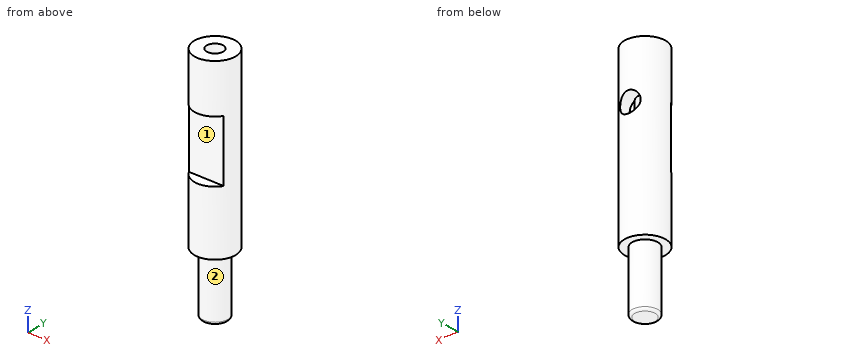
```python
from build123d import *

# Parameters (mm, degrees)
SKETCH1_R                      = 2.5
BOSS_EXTRUDE1_DEPTH            = 12
SKETCH2_R                      = 4
BOSS_EXTRUDE2_DEPTH            = 34
F_3_2_3_2_DIAMETER_HOLE1_D     = 3.2
F_3_2_3_2_DIAMETER_HOLE1_DEPTH = 13.03862301
F_3_2_3_2_DIAMETER_HOLE1_TIP   = 0.96137699
CUT_EXTRUDE1_DEPTH             = 35.467375879
CUT_EXTRUDE1_DEPTH_BACK        = 35.467375879
SKETCH6_W                      = 12
SKETCH6_H                      = 2
F_4_0_4_DIAMETER_HOLE3_D       = 4
F_4_0_4_DIAMETER_HOLE3_DEPTH   = 2.798278762
F_4_0_4_DIAMETER_HOLE3_TIP     = 1.201721238
FILLET1_R                      = 0.5


with BuildPart() as part:
    # Sketch1 → Boss-Extrude1 (new body)
    with BuildSketch(Plane.XY):
        Circle(SKETCH1_R)
    extrude(amount=-BOSS_EXTRUDE1_DEPTH)

    # Sketch2 → Boss-Extrude2 (add)
    with BuildSketch(Plane.XY):
        Circle(SKETCH2_R)
    extrude(amount=BOSS_EXTRUDE2_DEPTH)

    # Ø3.2 (3.2) Diameter Hole1
    with Locations(Plane.XY.offset(34)):
        with Locations((0, 0)):
            Hole(F_3_2_3_2_DIAMETER_HOLE1_D / 2, depth=F_3_2_3_2_DIAMETER_HOLE1_DEPTH)
            with Locations((0, 0, -(F_3_2_3_2_DIAMETER_HOLE1_DEPTH + F_3_2_3_2_DIAMETER_HOLE1_TIP / 2))):  # 118° drill point
                Cone(0, F_3_2_3_2_DIAMETER_HOLE1_D / 2, F_3_2_3_2_DIAMETER_HOLE1_TIP, mode=Mode.SUBTRACT)

    # Sketch6 → Cut-Extrude1 (cut, two sides: drawn at the far end of the back side and taken through both)
    with BuildSketch(Plane(origin=(0, 0, 0), x_dir=(0, 0, -1), z_dir=(1, 0, 0)).offset(-CUT_EXTRUDE1_DEPTH_BACK)):
        with Locations((-18.5, -3)):
            Rectangle(SKETCH6_W, SKETCH6_H)
    extrude(amount=CUT_EXTRUDE1_DEPTH + CUT_EXTRUDE1_DEPTH_BACK, mode=Mode.SUBTRACT)

    # Ø4.0 (4) Diameter Hole3
    with Locations(Plane(origin=(-0.101557348, 3.998710555, 23.218070674), x_dir=(0.999677638825, 0.025389337009, 0), z_dir=(-0.025389337009, 0.999677638825, 0))):
        with Locations((0, 0)):
            Hole(F_4_0_4_DIAMETER_HOLE3_D / 2, depth=F_4_0_4_DIAMETER_HOLE3_DEPTH)
            with Locations((0, 0, -(F_4_0_4_DIAMETER_HOLE3_DEPTH + F_4_0_4_DIAMETER_HOLE3_TIP / 2))):  # 118° drill point
                Cone(0, F_4_0_4_DIAMETER_HOLE3_D / 2, F_4_0_4_DIAMETER_HOLE3_TIP, mode=Mode.SUBTRACT)

    # Fillet1
    fillet1_edges = [part.edges().sort_by_distance(p)[0] for p in [
        (-2.5, 0, -12),
    ]]
    fillet(fillet1_edges, radius=FILLET1_R)


solid = part.part
```
Geometry check sheet. Reference: the model listing, model coordinates, mm. Face numbers are marked on the shaded views. Give positions to 0.01 mm unless a question says otherwise; leave off trailing zeros. Order: outer loops, then holes, each group sorted by start corner. A loop starts at its lowest first (then second) coordinate and runs counter-clockwise, first axis right, second up.
1. Section check D-D, the plane z = 4.5. Enter the section's corners in (x, y).
2. Thickness scan on L1, parallel to Y at x = 0, z = 26.5; L2, parallel to Y at x = -1.5, z = -6; L3, parallel to Z at x = 3, y = 1.75. Record the ranges inside material, lowest first.
3. Gauge pin test, flat ends, axial feed: pin 1 Ø0.6 at (x, y) = (-0.5, -3.5) entering from -Z; pin 2 Ø1 at (y, z) = (-1, 17.5) entering from +X; pin 3 Ø2.5 at (x, y) = (0, 0) entering from +Z. Record the tip position at first contact, or that the pin passes through.
4. Release check for a two-part mould opening along Z. For the marked faces 1 and 2 record: pulls with the +Z half, pulls with the -Z half, needs draft (parallel to the pull), parting line crosses it, or undercut.
5. Section check B-B, the plane z = 19.5. Enter the section's corners in (x, y), and give its area (3 significant figures).
6. Section check A-A, the plane y = -3.25. Enter the section's corners in (x, z), and give its area (3 significant figures).
7. Section check C-C, the plane z = -4. Enter the section's corners in (x, y).
Values follow:
1. outline: circle Ø8 at (0, 0)
2. L1: y = -4 to -1.6, 1.6 to 4
2. L2: y = -2 to 2
2. L3: z = 0 to 34
3. pin 1: stops at z = 0
3. pin 2: stops at x = 3.97
3. pin 3: stops at z = 20.75
4. face 1: undercut
4. face 2: needs draft
5. outline: (-3.46, -2) - (3.46, -2) arc R4 ccw (long way) to start
5. area: 40.4 mm2
6. outline: (-2.33, 0) - (2.33, 0) - (2.33, 12.5) - (-2.33, 12.5) - close; (-2.33, 24.5) - (2.33, 24.5) - (2.33, 34) - (-2.33, 34) - close
6. area: 103 mm2
7. outline: circle Ø5 at (0, 0)
